For this review, take the finished solid that the model builds, in its own axes (mm). Face numbers are marked on the shaded views. A direction names the side the tool comes from. Round coordinates to 2 decimals unless told otherwise and drop trailing zeros. Loops run counter-clockwise (first coordinate to the right, second up) from the corner with the lowest first, then second, coordinate; pieces in that order, holes last.
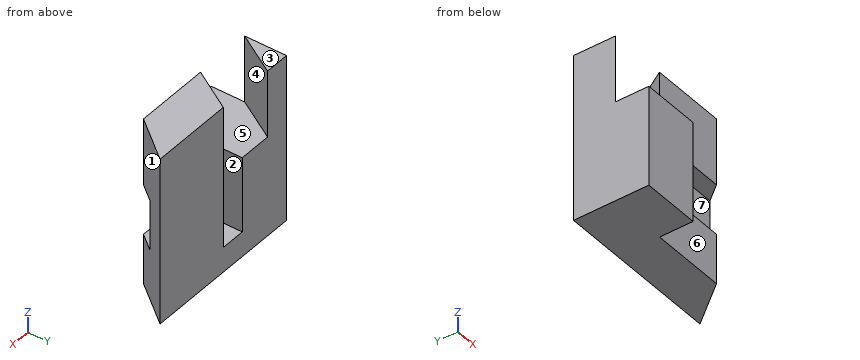
```python
from build123d import *

# Parameters (mm, degrees)
F0_W      = 100
F0_H      = 100
F1_DEPTH  = 45
F2_W      = 65
F2_H      = 20
F3_DEPTH  = 100
F5_DEPTH  = 100
F7_DEPTH  = 40
F10_DEPTH = 85
F11_W     = 14.643555
F11_H     = 30
F11_W_2   = 22.142187
F12_DEPTH = 10


with BuildPart() as f1:
    # F0 (on Front) → F1 (new body)
    with BuildSketch(Plane.XZ):
        with Locations((-50, 50)):
            Rectangle(F0_W, F0_H)
    extrude(amount=F1_DEPTH)

    # F2 (on face) → F3 (cut, through all)
    with BuildSketch(Plane.XY.offset(100)):
        with Locations((-32.5, -35)):
            Rectangle(F2_W, F2_H)
    extrude(amount=-F3_DEPTH, mode=Mode.SUBTRACT)

    # F4 (on face) → F5 (cut, through all)
    with BuildSketch(Plane.XY.offset(100)):
        Polygon((0, -25), (0, 0), (-20, -25), align=None)
    extrude(amount=-F5_DEPTH, mode=Mode.SUBTRACT)

    # F2 (on face) → F7 (cut, through all)
    with BuildSketch(Plane.XY.offset(100)):
        Polygon((-65, 0), (-85, 0), (-100, -25), (-100, -45), (-65, -45), (-65, -25), align=None)
    extrude(amount=-F7_DEPTH, mode=Mode.SUBTRACT)

    # F8 (on face) → F10 (cut, through all)
    with BuildSketch(Plane.XY.offset(100)):
        Polygon((-50, 0), (-65, 0), (-65, -24.8), align=None)
    extrude(amount=-F10_DEPTH, mode=Mode.SUBTRACT)

    # F11 (on face) → F12 (cut)
    with BuildSketch(Plane.XZ.offset(25)):
        with Locations((-12.678223, 45)):
            Rectangle(F11_W, F11_H)
        with Locations((-31.071093, 45)):
            Rectangle(F11_W_2, F11_H)
    extrude(amount=-F12_DEPTH, mode=Mode.SUBTRACT)


solid = f1.part
```
(1) For L1, parallel to X at y = -43, z = 22; L2, parallel to Y at x = -16.5, z = 43; L3, parallel to Z at x = -64, y = -1.5, list the stretches that pass through material, from the lowest coordinate up.
(2) For the marked faces 5, 6 and 7, list the 3-axis set-ups (+Z, -Z, +X, -X, +Y, -Y) from which the entire face can be reached by the end or side of a thin tool; tool diameter is ignored.
(3) Add section C-C (z = 35). Give the boundary of the cut face in (x, y).
(4) Add section A-A (z = 77). Give the boundary of the cut face in (x, y), plus the area to 3 significant figures.
(5) The part is to be moulded in two halves that separate along X. For the marked faces 1, 2, 3 and 4, say which applies: pulls with the +X half, pulls with the -X half, needs draft (parallel to the pull), parting line crosses it, or undercut.
(6) Add section B-B (x = -37.5). Give the boundary of the cut face in (y, z).
(7) Insertion check: pin 1 Ø6 at (y, z) = (-34, 23) entering from +X; pin 2 Ø2 at (y, z) = (-14.5, 75.5) entering from +X; pin 3 Ø1.5 at (y, z) = (-25, 28.5) entering from +X. Each pin has a flat end and moves straight along its axis. Give the tip position at first contact, or say it passes through.
(8) Add section D-D (y = -4.5). Give the boundary of the cut face in (x, z), plus the area to 3 significant figures.
Outcome:
1. L1: x = -100 to -65
1. L2: y = -15 to 0
1. L3: z = 0 to 15
2. face 5: +Z, -Y
2. face 6: +Z, -Z, +X, -Y
2. face 7: +X, -Y
3. outline: (-100, -45) - (-65, -45) - (-65, -25) - (-42.14, -25) - (-42.14, -15) - (-12, -15) - (0, 0) - (-50, 0) - (-65, -24.8) - (-65, 0) - (-100, 0) - close
4. outline: (-100, -25) - (-85, 0) - (-100, 0) - close; (-65, -25) - (-20, -25) - (0, 0) - (-50, 0) - (-65, -24.8) - close
4. area: 1,380 mm2
5. face 1: pulls with the +X half
5. face 2: undercut
5. face 3: needs draft
5. face 4: undercut
6. outline: (-25, 0) - (0, 0) - (0, 100) - (-25, 100) - (-25, 60) - (-15, 60) - (-15, 30) - (-25, 30) - close
7. pin 1: stops at x = -65
7. pin 2: stops at x = -10.8
7. pin 3: stops at x = -19.4
8. outline: (-100, 0) - (-3.6, 0) - (-3.6, 100) - (-52.72, 100) - (-52.72, 15) - (-65, 15) - (-65, 60) - (-87.7, 60) - (-87.7, 100) - (-100, 100) - close
8. area: 7,690 mm2
